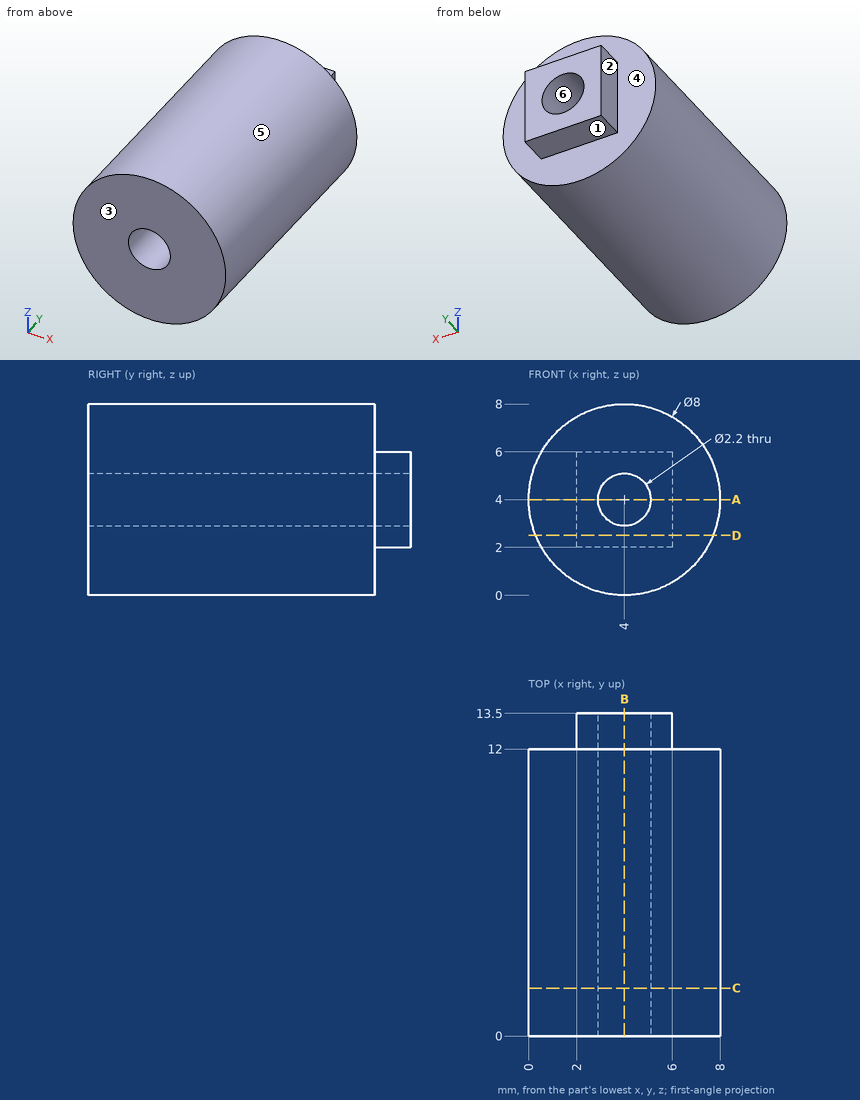
Check sheet for the drawn part. Datum: minimum x, y, z corner. Units: mm. A direction names the side the tool comes from. Round coordinates to 2 decimals unless told otherwise and drop trailing zeros. Write each loop counter-clockwise with the first axis right and the second up, starting at its lowest first coordinate (ties: lowest second). Pieces come first, ordered by that corner, then holes. Notation, with made-up numbers: (-18.5, -10.75) -> (26.5, -10.75) arc R35 ccw to (26.5, 27.25) -> close; hole circle Ø8 at (-30, 17.25). An arc over 180 degrees is marked (long way). One line per item, written item: value. Start each with the question number.
(1) Cross-section at C-C, the plane y = 2. Record the cut outline in (x, z), and give its area (3 significant figures).
(2) Go/stop test with flat-tipped pins: pin 1 Ø2 at (x, y) = (6.5, 6.5) entering from -Z; pin 2 Ø1.6 at (y, z) = (13, 3.5) entering from +X; pin 3 Ø1.5 at (y, z) = (7, 6.5) entering from +X; pin 4 Ø2 at (x, z) = (4, 4) entering from -Y. Record where each tip stops, or that it passes through.
(3) Scan lines: line 1 (Z direction, x = 4, y = 4); line 2 (Y direction, x = 5.25, z = 1.5); line 3 (X direction, y = 8.75, z = 4.5). Record each from-to range of solid material in increasing order. Write a range as [from, to].
(4) Access from +Z, -Z, +X, -X, +Y, -Y to the whole of each face (thin tool, end or side, straight path). Record for the marked faces 1, 2 and 3.
(5) Draft check along X on the marked faces 4, 5 and 6. Enter one of: +X half, -X half, draft (parallel to the pull), parting line (faces both ways), or undercut.
(6) Cross-section at A-A, the plane z = 4. Record the cut outline in (x, y), and give its area (3 significant figures).
(7) Cross-section at B-B, the plane x = 4. Record the cut outline in (y, z), and give its area (3 significant figures).
(8) Cross-section at D-D, the plane z = 2.5. Record the cut outline in (x, y), and give its area (3 significant figures).
Answer:
1. outline: circle Ø8 at (4, 4); hole circle Ø2.2 at (4, 4)
1. area: 46.5 mm²
2. pin 1: z = 0.29
2. pin 2: x = 6
2. pin 3: x = 7.6
2. pin 4: through
3. line 1: [0, 2.9], [5.1, 8]
3. line 2: [0, 12]
3. line 3: [0.03, 3.02], [4.98, 7.97]
4. face 1: -Z, +X, -X, +Y
4. face 2: +Z, -Z, -X, +Y
4. face 3: +Z, -Z, +X, -X, -Y
5. face 4: draft
5. face 5: parting line
5. face 6: undercut
6. outline: (0, 0) -> (2.9, 0) -> (2.9, 13.5) -> (2, 13.5) -> (2, 12) -> (0, 12) -> close; (5.1, 0) -> (8, 0) -> (8, 12) -> (6, 12) -> (6, 13.5) -> (5.1, 13.5) -> close
6. area: 72.3 mm²
7. outline: (0, 0) -> (12, 0) -> (12, 2) -> (13.5, 2) -> (13.5, 2.9) -> (0, 2.9) -> close; (0, 5.1) -> (13.5, 5.1) -> (13.5, 6) -> (12, 6) -> (12, 8) -> (0, 8) -> close
7. area: 72.3 mm²
8. outline: (0.29, 0) -> (7.71, 0) -> (7.71, 12) -> (6, 12) -> (6, 13.5) -> (2, 13.5) -> (2, 12) -> (0.29, 12) -> close
8. area: 95.0 mm²
